For this review, take the finished solid that the model builds, in its own axes (mm). Face numbers are marked on the shaded views. A direction names the side the tool comes from. Round coordinates to 2 decimals unless told otherwise and drop trailing zeros. Order: outer loops, then holes, each group sorted by start corner. A loop starts at its lowest first (then second) coordinate and runs counter-clockwise, first axis right, second up. Notation, with made-up numbers: (58.5, 5.5) - (72.5, 5.5) arc R22 ccw to (72.5, 25.5) - close; hole circle Ø8 at (10, -6). An arc over 180 degrees is marked (long way). One line per item, written item: value.
```python
from build123d import *

# Parameters (mm, degrees)
F1_DEPTH = 15
F4_D     = 4.1
F4_DEPTH = 7
F5_D     = 6.1
F5_DEPTH = 7


with BuildPart() as f1:
    # F0 (on Top) → F1 (new body)
    with BuildSketch(Plane.XY):
        Polygon((-8.678603, 13), (-10.678603, 13), (-10.678603, -13.5), (16.421397, -13.5), (16.421397, 13), (11.421397, 13), (11.421397, -7.1), (6.971397, -7.1), (6.971397, -10.4), (-4.228603, -10.4), (-4.228603, -7.1), (-8.678603, -7.1), (-8.678603, 0), (-7.678603, 0), (-8.678603, 6), align=None)
    extrude(amount=F1_DEPTH)

    # F4
    with Locations(Plane.YZ.offset(16.421397)):
        with Locations((3, 7.5)):
            Hole(F4_D / 2, depth=F4_DEPTH)

    # F5
    with Locations(Plane.XZ.offset(13.5)):
        with Locations((1.371397, 7.5)):
            Hole(F5_D / 2, depth=F5_DEPTH)


solid = f1.part
```
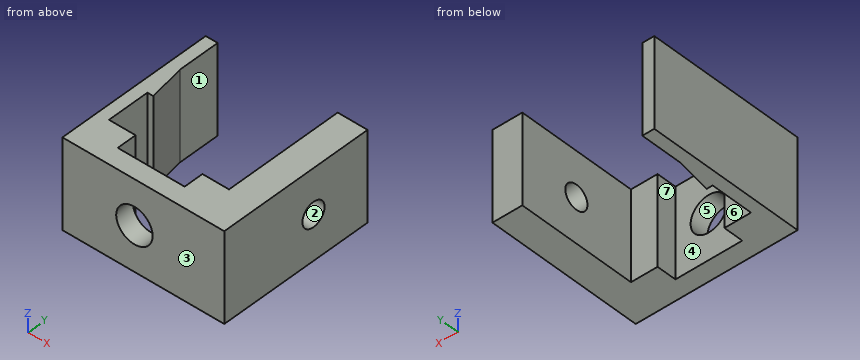
Item 1: Take a section at A-A (z = 7.5). Write out the cut boundary in (x, y), plus the area to 3 significant figures.
Returned:
outline: (-10.68, -13.5) - (-1.68, -13.5) - (-1.68, -10.4) - (-4.23, -10.4) - (-4.23, -7.1) - (-8.68, -7.1) - (-8.68, 0) - (-7.68, 0) - (-8.68, 6) - (-8.68, 13) - (-10.68, 13) - close; (4.42, -13.5) - (16.42, -13.5) - (16.42, 0.95) - (11.42, 0.95) - (11.42, -7.1) - (6.97, -7.1) - (6.97, -10.4) - (4.42, -10.4) - close; (11.42, 5.05) - (16.42, 5.05) - (16.42, 13) - (11.42, 13) - close
area: 241 mm^2
Item 2: Take a section at B-B (y = 6.5). Write out the cut boundary in (x, z).
Returned:
outline: (-10.68, 0) - (-8.68, 0) - (-8.68, 15) - (-10.68, 15) - close; (11.42, 0) - (16.42, 0) - (16.42, 15) - (11.42, 15) - close
Item 3: Take a section at C-C (x = 1). Write out the cut boundary in (y, z), plus the area to 3 significant figures.
Returned:
outline: (-13.5, 0) - (-10.4, 0) - (-10.4, 4.47) - (-13.5, 4.47) - close; (-13.5, 10.53) - (-10.4, 10.53) - (-10.4, 15) - (-13.5, 15) - close
area: 27.7 mm^2
Item 4: Wall thickness on line 1 (X direction, y = 10.5, z = 2.5); line 2 (X direction, y = -9.25, z = 4.5); line 3 (Z direction, x = 13.35, y = 3): over which ranges is each line inside the solid? List them lowest first.
Returned:
line 1: -10.68 to -8.68, 11.42 to 16.42
line 2: -10.68 to -4.23, 6.97 to 16.42
line 3: 0 to 5.45, 9.55 to 15
Item 5: Machinability: for the marked faces 5, 6 and 7, which of the approach directions +Z, -Z, +X, -X, +Y, -Y give a long, thin tool a straight path to every point of the face, cutting with its end or side? Answer none if there is none.
Returned:
face 5: +Y, -Y
face 6: +Z, -Z
face 7: +Z, -Z, +Y
Item 6: Take a section at D-D (y = 3). Write out the cut boundary in (x, z), plus the area to 3 significant figures.
Returned:
outline: (-10.68, 0) - (-8.18, 0) - (-8.18, 15) - (-10.68, 15) - close; (11.42, 0) - (16.42, 0) - (16.42, 5.45) - (11.42, 5.45) - close; (11.42, 9.55) - (16.42, 9.55) - (16.42, 15) - (11.42, 15) - close
area: 92.0 mm^2
Item 7: The part is to be moulded in two halves that separate along Y. For the marked faces 1, 2, 3 and 4, say which applies: +Y half, -Y half, draft (parallel to the pull), parting line (faces both ways), or undercut.
Returned:
face 1: draft
face 2: undercut
face 3: -Y half
face 4: +Y half
Item 8: For P1, Ø1.3, axis at x = 9.5, z = 8.5, coming from the +Y side, flat-tipped, find the tip position at first contact; note if it passes through.
Returned:
P1: y = -7.1
